Geometry check sheet. Reference: the model listing, model coordinates, mm. A direction names the side the tool comes from. Give positions to 0.01 mm unless a question says otherwise; leave off trailing zeros. Write each loop counter-clockwise with the first axis right and the second up, starting at its lowest first coordinate (ties: lowest second). Pieces come first, ordered by that corner, then holes. Notation, with made-up numbers: (-31.5, 89) - (9.5, 89) arc R28 ccw to (9.5, 120) - close; hole circle Ø3 at (-9, -37.75). An arc over 180 degrees is marked (long way). Write item = value, one per line. Start each with the question number.
(1) Section check B-B, the plane z = 106.5. Enter the section's corners in (x, y).
(2) Access from +Z, -Z, +X, -X, +Y, -Y to the whole of each face (thin tool, end or side, straight path). Record for faces 5 (the flat face through (-1, 38.1, 75)), 6 (the flat face through (51, -12.7, 13)), 7 (the flat face through (-1, 12.7, 74)).
(3) Depth check by flat-ended pin: pin 1 Ø7.5 at (x, z) = (51, 10) entering from -Y; pin 2 Ø3 at (x, y) = (-9.5, 2.5) entering from +Z; pin 3 Ø12.5 at (y, z) = (-27, 11.5) entering from +X. Enter the tip coordinate at first touch or a pass-through.
(4) Draft check along Z on faces 1 (the cylindrical face through (-44.405, 25.578, 134.292)), 2 (the flat face through (-63.5, 16, 34)), 3 (the cylindrical face through (-5.75, 25.22, 76.83)), 4 (the flat face through (-1, 1, 0)). Enter one of: pulls with the +Z half, pulls with the -Z half, needs draft (parallel to the pull), parting line crosses it, or undercut.
(5) Section check C-C, the plane y = 1. Enter the section's corners in (x, z).
(6) Section check A-A, the plane x = -4. Enter the section's corners in (y, z), plus the area to 3 significant figures.
(7) Section check D-D, the plane z = 33.5. Enter the section's corners in (x, y).
(8) Thickness scan on L1, parallel to Z at x = -34, y = -18.5; L2, parallel to Y at x = 19.5, z = 144.5; L3, parallel to X at y = 32, z = 91.5. Record the ranges inside material, lowest first.
```python
from build123d import *

# Parameters (mm, degrees)
F1_DEPTH = 25.4
F2_W     = 127
F2_H     = 25.4
F3_DEPTH = 127
F4_R     = 63.5
F5_R     = 63.49999
F6_R     = 26.5461499869
F7_DEPTH = 25.401


# Not quite as in the source:
# - a fillet or chamfer is up to 0.001 mm smaller than in the source, because OpenCascade refuses the exact size


with BuildPart() as f1:
    # F0 (on Top) → F1 (new body)
    with BuildSketch(Plane.XY):
        Polygon((63.5, -12.7), (63.5, 38.1), (-63.5, 38.1), (-63.5, -38.1), (38.1, -38.1), (38.1, -12.7), align=None)
    extrude(amount=F1_DEPTH)

    # F2 (on face) → F3 (join)
    with BuildSketch(Plane.XY.offset(25.4)):
        with Locations((0, 25.4)):
            Rectangle(F2_W, F2_H)
    extrude(amount=F3_DEPTH)

    # F4
    f4_edges = [f1.edges().sort_by_distance(p)[0] for p in [
        (63.5, 25.4, 152.4),
    ]]
    fillet(f4_edges, radius=F4_R)

    # F5 (radius 63.5 in the source; OpenCascade refuses exactly that, so slightly less here)
    f5_edges = [f1.edges().sort_by_distance(p)[0] for p in [
        (-63.5, 25.4, 152.4),
    ]]
    fillet(f5_edges, radius=F5_R)

    # F6 (on face) → F7 (cut, through all)
    with BuildSketch(Plane.XZ.offset(-12.7)):
        with Locations((0, 102.7461499869)):
            Circle(F6_R)
    extrude(amount=-F7_DEPTH, mode=Mode.SUBTRACT)


solid = f1.part
```
Model answer:
q1.outline = (-61.01, 12.7) - (-26.28, 12.7) - (-26.28, 38.1) - (-61.01, 38.1) - close; (26.28, 12.7) - (61.01, 12.7) - (61.01, 38.1) - (26.28, 38.1) - close
q2.face_5 = +Z, -Z, +X, -X, +Y
q2.face_6 = +Z, -Z, +X, -Y
q2.face_7 = +Z, +X, -X, -Y
q3.pin_1 = -12.7
q3.pin_2 = 25.4
q3.pin_3 = 38.1
q4.face_1 = pulls with the +Z half
q4.face_2 = needs draft
q4.face_3 = undercut
q4.face_4 = pulls with the -Z half
q5.outline = (-63.5, 0) - (63.5, 0) - (63.5, 25.4) - (-63.5, 25.4) - close
q6.outline = (-38.1, 0) - (38.1, 0) - (38.1, 76.5) - (12.7, 76.5) - (12.7, 25.4) - (-38.1, 25.4) - close; (12.7, 128.99) - (38.1, 128.99) - (38.1, 152.27) - (12.7, 152.27) - close
q6.area = 3,820 mm²
q7.outline = (-63.5, 12.7) - (63.5, 12.7) - (63.5, 38.1) - (-63.5, 38.1) - close
q8.L1 = 0 to 25.4
q8.L2 = 12.7 to 38.1
q8.L3 = -63.45 to -24.05, 24.05 to 63.45
